Study the drawing (mm; zero at the part's minimum x, y, z) and answer. Round coordinates to 2 decimals unless told otherwise and drop trailing zeros. Write each loop counter-clockwise with the first axis right and the second up, starting at its lowest first coordinate (ties: lowest second). Pieces come first, ordered by that corner, then holes. Notation, with made-up numbers: (10.25, 39.25) - (36.25, 39.25) arc R32 ccw to (36.25, 71.25) - close; hole circle Ø9 at (44, 40). An arc over 180 degrees is marked (long way). Return JSON: item names as keys, results as strings. Group by question number.
(1) Determine the mould class of the marked faces 1 and 2 for opening direction Y: +Y half, -Y half, draft (parallel to the pull), parting line (faces both ways), or undercut.
(2) Section C-C, the plane z = 6 is taken. Write down the section's boundary in (x, y), then the cut area to 3 significant figures.
(3) Each of these flat-tipped pins is pushed along its axis until it touches: pin 1 (2.5 mm diameter, centred on x = 66.5, z = 6.5, fed in from -Y); pin 2 (3 mm diameter, centred on x = 62, y = 3.5, fed in from +Z); pin 3 (4 mm diameter, centred on y = 33, z = 7.5, fed in from -X); pin 4 (1.5 mm diameter, centred on x = 90.5, z = 7, fed in from +Y). Where does it stop, or does it pass through?
(4) Section B-B, the plane y = 32 is taken. Write down the section's boundary in (x, z).
(5) Find the intervals of material crossed by line 1 along X through (y, z) = (34, 5.75); line 2 along Y through (x, z) = (34.5, 5.75); line 3 along Z through (x, y) = (74, 6.5), in increasing order. Write a range as [from, to].
(6) Section A-A, the plane x = 133.5 is taken. Write down the section's boundary in (y, z).
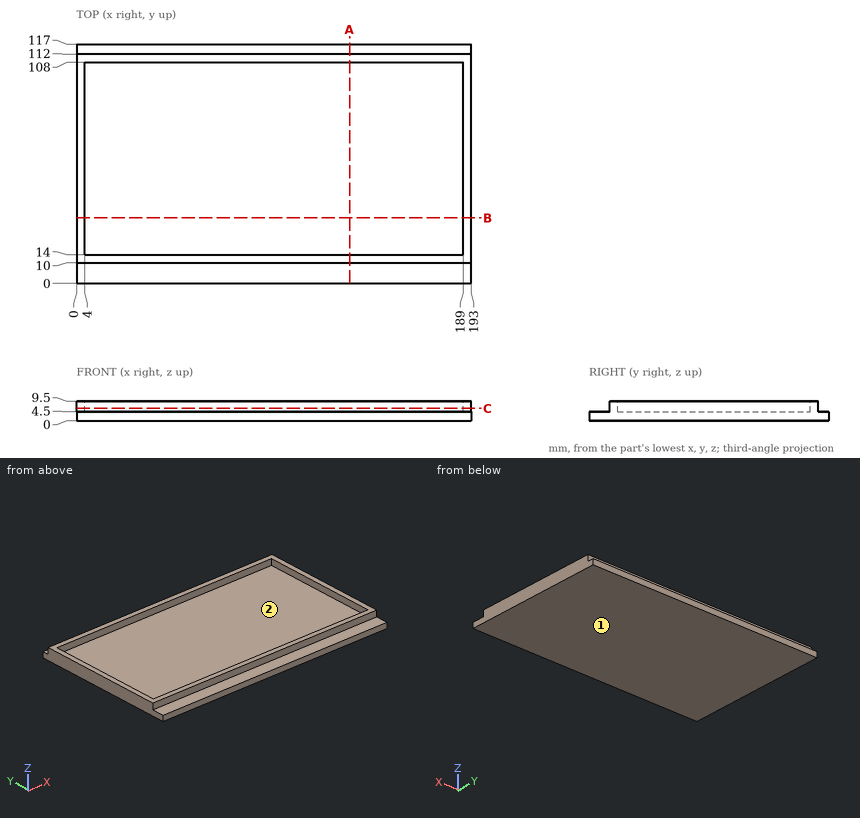
Working result:
{
 "1": {"face 1": "draft", "face 2": "undercut"},
 "2": {"outline": "(0, 10) - (193, 10) - (193, 112) - (0, 112) - close; hole (4, 14) - (189, 14) - (189, 108) - (4, 108) - close", "area": "2,300 mm^2"},
 "3": {"pin 1": "stops at y = 10", "pin 2": "stops at z = 4.5", "pin 3": "stops at x = 0", "pin 4": "stops at y = 112"},
 "4": {"outline": "(0, 0) - (193, 0) - (193, 9.5) - (189, 9.5) - (189, 4.5) - (4, 4.5) - (4, 9.5) - (0, 9.5) - close"},
 "5": {"line 1": "x = [0, 4], [189, 193]", "line 2": "y = [10, 14], [108, 112]", "line 3": "z = [0, 4.5]"},
 "6": {"outline": "(0, 0) - (117, 0) - (117, 4.5) - (112, 4.5) - (112, 9.5) - (108, 9.5) - (108, 4.5) - (14, 4.5) - (14, 9.5) - (10, 9.5) - (10, 4.5) - (0, 4.5) - close"}
}
